from build123d import *

# Parameters (mm, degrees)
SKETCH013_W            = 190
SKETCH013_H            = 112
PAD009_DEPTH           = 20
SKETCH014_W            = 180
SKETCH014_H            = 50
POCKET004_DEPTH        = 14
SKETCH015_W            = 187
SKETCH015_H            = 28
POCKET005_DEPTH        = 18.5
LINEARPATTERN007_COUNT = 2
LINEARPATTERN007_PITCH = 29.5
FILLET013_R            = 3
POCKET006_DEPTH        = 4.5
FILLET014_R            = 4
FILLET016_R            = 2


with BuildPart() as part:
    # Sketch013 → Pad009 (new body)
    with BuildSketch(Plane.XY):
        Rectangle(SKETCH013_W, SKETCH013_H)
    extrude(amount=PAD009_DEPTH)

    # Sketch014 (on DatumPlane) → Pocket004 (cut)
    with BuildSketch(Plane(origin=(0, 4.5, 20), x_dir=(1, 0, 0), z_dir=(0, 0, 1))):
        with Locations((0, 25)):
            Rectangle(SKETCH014_W, SKETCH014_H)
    extrude(amount=-POCKET004_DEPTH, mode=Mode.SUBTRACT)

    # Sketch015 (on DatumPlane) → Pocket005 (cut)
    with BuildSketch(Plane(origin=(0, 3, 20), x_dir=(1, 0, 0), z_dir=(0, 0, 1))):
        with Locations((0, -14)):
            Rectangle(SKETCH015_W, SKETCH015_H)
    pocket005 = extrude(amount=-POCKET005_DEPTH, mode=Mode.SUBTRACT)

    # LinearPattern007: Pocket005 ×2
    with Locations(*[(0, -i * LINEARPATTERN007_PITCH, 0) for i in range(1, LINEARPATTERN007_COUNT)]):
        add(pocket005, mode=Mode.SUBTRACT)

    # Fillet013
    fillet013_edges = [part.edges().sort_by_distance(p)[0] for p in [
        (93.5, 3, 10.75),
        (93.5, -26.5, 10.75),
        (-93.5, 3, 10.75),
        (-93.5, -26.5, 10.75),
        (-93.5, -25, 10.75),
        (-93.5, -54.5, 10.75),
        (93.5, -25, 10.75),
        (93.5, -54.5, 10.75),
    ]]
    fillet(fillet013_edges, radius=FILLET013_R)

    # Sketch016 (on DatumPlane) → Pocket006 (cut)
    with BuildSketch(Plane(origin=(0, 4.5, 6), x_dir=(1, 0, 0), z_dir=(0, 0, 1))):
        with BuildLine():
            ThreePointArc((-85.299989, 28.479983), (-88.479983, 14.700011), (-74.700011, 11.520017))
            Line((-74.700011, 11.520017), (-42.700011, 31.520017))
            ThreePointArc((-42.700011, 31.520017), (-39.520017, 45.299989), (-53.299989, 48.479983))
            Line((-53.299989, 48.479983), (-85.299989, 28.479983))
        make_face()
    pocket006 = extrude(amount=-POCKET006_DEPTH, mode=Mode.SUBTRACT)

    # Mirrored002: Pocket006 across Sketch016 V_Axis
    add(pocket006.mirror(Plane(origin=(0, 4.5, 6), x_dir=(0, 0, 1), z_dir=(1, 0, 0))), mode=Mode.SUBTRACT)

    # Fillet014
    fillet014_edges = [part.edges().sort_by_distance(p)[0] for p in [
        (88.479983, 19.200011, 1.5),
        (58.700011, 26.020017, 1.5),
        (39.520017, 49.799989, 1.5),
        (69.299989, 42.979983, 1.5),
        (-88.479983, 19.200011, 1.5),
        (-58.700011, 26.020017, 1.5),
        (-39.520017, 49.799989, 1.5),
        (-69.299989, 42.979983, 1.5),
    ]]
    fillet(fillet014_edges, radius=FILLET014_R)

    # Fillet016
    fillet016_edges = [part.edges().sort_by_distance(p)[0] for p in [
        (0, 56, 0),
        (95, 0, 0),
        (0, -56, 0),
        (-95, 0, 0),
        (-95, -56, 10),
        (-95, 56, 10),
        (95, 56, 10),
        (95, -56, 10),
    ]]
    fillet(fillet016_edges, radius=FILLET016_R)


with BuildPart() as part_1:
    # Body004 placement: moved
    add(part.part.moved(Location((0, -20, 0))))


solid = part_1.part
Can you work these out from the model? Positions are in its coordinate system, mm. A direction names the side the tool comes from. Give positions to 0.01 mm unless a question says otherwise; leave off trailing zeros. Write each loop counter-clockwise with the first axis right and the second up, starting at its lowest first coordinate (ties: lowest second). Pieces come first, ordered by that corner, then holes. Notation, with made-up numbers: M 25,24.5 L 39,24.5 A20 cw 39,41.5 Z; hole C 87,-0.75 d8. An arc over 180 degrees is marked long. Answer in a Markdown table with one row per item. Add a question column.
Item 1: Imagine slicing it at B-B, the plane y = -27. Write out the boundary of the cut face in (x, z).
Item 2: Imagine slicing it at A-A, the plane z = 15. Write out the boundary of the cut face in (x, y), plus the area to 3 significant figures.
Item 3: We'd pull the mould along X, two halves only. Please class faces 1 (the flat face through (-1, -74.5, 11)), 2 (the flat face through (-1, -76, 11)): released by +X, released by -X, zero draft, split by the parting line, or undercut.
Item 4: For pin 1 Ø6 at (x, y) = (71, -39) entering from +Z; pin 2 Ø16 at (x, y) = (-57.5, 10.5) entering from +Z, each with a flat end and sliding along its axis, tell me the tip position at first contact or that it passes through.
Item 5: Imagine slicing it at C-C, the plane x = -22. Write out the boundary of the cut face in (y, z), plus the area to 3 significant figures.
Item 6: Please list where these lines run through material, in increasing order: L1, parallel to Y at x = -1.5, z = 7.5; L2, parallel to Y at x = -38, z = 3; L3, parallel to X at y = -39.5, z = 10.75.
Item 7: On a 3-axis mill with a long thin cutter (end or side, diameter ignored), from which of +Z, -Z, +X, -X, +Y, -Y can I reach the whole of each face in a straight line? I mean faces 3 (the flat face through (-1, -19, 0)), 4 (the flat face through (-1, -60, 1.5)). Say none if no direction works.
Evaluation:
| question | item | result |
|---|---|---|
| 1 | outline | M -95,2 A2 ccw -93,0 L 93,0 A2 ccw 95,2 L 95,20 L 93.5,20 L 93.5,1.5 L -93.5,1.5 L -93.5,20 L -95,20 Z |
| 2 | outline | M -95,-74 A2 ccw -93,-76 L 93,-76 A2 ccw 95,-74 L 95,34 A2 ccw 93,36 L -93,36 A2 ccw -95,34 Z; hole M -93.5,-71.5 A3 ccw -90.5,-74.5 L 90.5,-74.5 A3 ccw 93.5,-71.5 L 93.5,-49.5 A3 ccw 90.5,-46.5 L -90.5,-46.5 A3 ccw -93.5,-49.5 Z; hole M -93.5,-42 A3 ccw -90.5,-45 L 90.5,-45 A3 ccw 93.5,-42 L 93.5,-20 A3 ccw 90.5,-17 L -90.5,-17 A3 ccw -93.5,-20 Z; hole M -90,-15.5 L 90,-15.5 L 90,34.5 L -90,34.5 Z |
| 2 | area | 1,820 mm² |
| 3 | face 1 | undercut |
| 3 | face 2 | zero draft |
| 4 | pin 1 | stops at z = 1.5 |
| 4 | pin 2 | stops at z = 6 |
| 5 | outline | M -76,2 A2 ccw -74,0 L 34,0 A2 ccw 36,2 L 36,20 L 34.5,20 L 34.5,6 L -15.5,6 L -15.5,20 L -17,20 L -17,1.5 L -45,1.5 L -45,20 L -46.5,20 L -46.5,1.5 L -74.5,1.5 L -74.5,20 L -76,20 Z |
| 5 | area | 502 mm² |
| 6 | L1 | y = -76 to -74.5, -46.5 to -45, -17 to -15.5, 34.5 to 36 |
| 6 | L2 | y = -76 to -74.5, -46.5 to -45, -17 to 36 |
| 6 | L3 | x = -95 to -93.5, 93.5 to 95 |
| 7 | face 3 | -Z, +X, -X, +Y, -Y |
| 7 | face 4 | +Z |
